Verification items for the finished model (mm, model axes). A direction names the side the tool comes from. Give positions to 0.01 mm unless a question says otherwise; leave off trailing zeros. Order: outer loops, then holes, each group sorted by start corner. A loop starts at its lowest first (then second) coordinate and runs counter-clockwise, first axis right, second up. Notation, with made-up numbers: (55.5, 5.5) -> (65.5, 5.5) arc R14 ccw to (65.5, 10.5) -> close; hole circle Ø3 at (35, 17.25). An arc over 180 degrees is marked (long way). Return JSON: item names as keys, results as strings. Group by question number.
(1) Cross-section at A-A on y = 0. Enter the section's corners in (x, z) (1 decimal), then the cut area to 3 significant figures.
(2) Depth check by flat-ended pin: pin 1 Ø8 at (x, y) = (-106, -7.5) entering from +Z; pin 2 Ø1 at (x, y) = (-287, 11.5) entering from -Z; pin 3 Ø6 at (x, z) = (-64.5, -17) entering from +Y; pin 4 Ø21.5 at (y, z) = (13, 4.5) entering from -X. Enter the tip coordinate at first touch or a pass-through.
(3) Release check for a two-part mould opening along Y. For faces 3 (the face through (-212.88, -36.76, 8.16)), 4 (the face through (-199.479, -21.251, 27.715)), 5 (the face through (0, -25, -25)) record: pulls with the +Y half, pulls with the -Y half, needs draft (parallel to the pull), parting line crosses it, or undercut.
(4) Thickness scan on line 1 along Y through (x, z) = (-405.2, 0); line 2 along Y through (x, z) = (-426, 0) (1 decimal); line 3 along Z through (x, y) = (-136.5, -11). Record the ranges inside material, lowest first.
(5) Cross-section at B-B on z = 14. Enter the section's corners in (x, y).
(6) Tool access check on faces 1 (the face through (-418.523, -21.251, 27.715)), 2 (the face through (-404.622, -7.8, 34.4)). Record the directions out of +Z, -Z, +X, -X, +Y, -Y that give a thin tool (end or side, any length) a straight path to the whole face; none if there is none.
from build123d import *

# Parameters (mm, degrees)
SKETCH1_R           = 37.6555
SKETCH1_R_2         = 34.925
BOSS_EXTRUDE1_DEPTH = 431.8
SKETCH3_W           = 0.9906
SKETCH3_H           = 0.9652


with BuildPart() as part:
    # Sketch1 → Boss-Extrude1 (new body)
    with BuildSketch(Plane(origin=(0, 0, 0), x_dir=(0, 0, -1), z_dir=(1, 0, 0))):
        Circle(SKETCH1_R)
        Circle(SKETCH1_R_2, mode=Mode.SUBTRACT)
    extrude(amount=-BOSS_EXTRUDE1_DEPTH)

    # Sketch3 → Z-92479A230 Snap Ring Groove (revolve, cut)
    with BuildSketch(Plane.XY, mode=Mode.PRIVATE) as z_92479a230_snap_ring_groove_sk:
        with Locations((-405.1173, 35.4076)):
            Rectangle(SKETCH3_W, SKETCH3_H)
    revolve(z_92479a230_snap_ring_groove_sk.sketch.rotate(Axis((-431.8, 0, 0), (1, 0, 0)), 270), axis=Axis((-431.8, 0, 0), (1, 0, 0)), mode=Mode.SUBTRACT)


solid = part.part
Verdict:
{
 "1": {"outline": "(-431.8, -37.7) -> (0, -37.7) -> (0, -34.9) -> (-404.6, -34.9) -> (-404.6, -35.9) -> (-405.6, -35.9) -> (-405.6, -34.9) -> (-431.8, -34.9) -> close; (-431.8, 34.9) -> (-405.6, 34.9) -> (-405.6, 35.9) -> (-404.6, 35.9) -> (-404.6, 34.9) -> (0, 34.9) -> (0, 37.7) -> (-431.8, 37.7) -> close", "area": "2,360 mm²"},
 "2": {"pin 1": "z = 37.49", "pin 2": "z = -36.01", "pin 3": "y = 34.96", "pin 4": "through"},
 "3": {"face 3": "parting line crosses it", "face 4": "undercut", "face 5": "needs draft"},
 "4": {"line 1": "-37.66 to -35.89, 35.89 to 37.66", "line 2": "-37.7 to -34.9, 34.9 to 37.7", "line 3": "-36.01 to -33.15, 33.15 to 36.01"},
 "5": {"outline": "(-431.8, -34.96) -> (0, -34.96) -> (0, -32) -> (-404.62, -32) -> (-404.62, -33.05) -> (-405.61, -33.05) -> (-405.61, -32) -> (-431.8, -32) -> close; (-431.8, 32) -> (-405.61, 32) -> (-405.61, 33.05) -> (-404.62, 33.05) -> (-404.62, 32) -> (0, 32) -> (0, 34.96) -> (-431.8, 34.96) -> close"},
 "6": {"face 1": "+X, -X", "face 2": "none"}
}
